For this review, take the finished solid that the model builds, in its own axes (mm). Face numbers are marked on the shaded views. Round coordinates to 2 decimals unless told otherwise and drop trailing zeros. Order: outer loops, then holes, each group sorted by start corner. A loop starts at its lowest first (then second) coordinate and runs counter-clockwise, first axis right, second up.
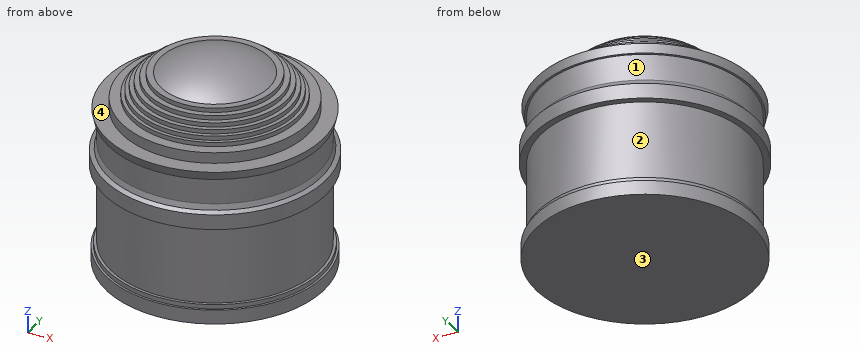
from build123d import *


with BuildPart() as f1:
    # F0 (on Front) → F1 (revolve)
    with BuildSketch(Plane.XZ):
        with BuildLine():
            Line((0, 76.2), (0, 38.1))
            Line((0, 38.1), (0, -76.2))
            Line((0, -76.2), (79.872511, -76.2))
            Line((79.872511, -76.2), (79.872511, -65.777272))
            Line((79.872511, -65.777272), (78.254335, -65.777272))
            Line((78.254335, -65.777272), (78.254335, -62.504791))
            Line((78.254335, -62.504791), (76.2, -62.504791))
            Line((76.2, -62.504791), (76.2, -4.198033))
            Line((76.2, -4.198033), (80.9625, -4.198033))
            Line((80.9625, -4.198033), (80.9625, 6.914467))
            Line((80.9625, 6.914467), (77.836014, 8.487052))
            Line((77.836014, 8.487052), (76.2, 12.349062))
            Line((76.2, 12.349062), (76.2, 31.75))
            Line((76.2, 31.75), (77.7875, 31.75))
            Line((77.7875, 31.75), (79.375, 38.1))
            Line((79.375, 38.1), (68.2625, 38.1))
            Line((68.2625, 38.1), (68.2625, 46.0375))
            Line((68.2625, 46.0375), (60.720578, 46.0375))
            Line((60.720578, 46.0375), (60.720578, 49.2125))
            Line((60.720578, 49.2125), (58.177056, 49.2125))
            Line((58.177056, 49.2125), (58.177056, 52.3875))
            Line((58.177056, 52.3875), (55.33525, 52.3875))
            Line((55.33525, 52.3875), (55.33525, 55.5625))
            Line((55.33525, 55.5625), (52.146415, 55.5625))
            Line((52.146415, 55.5625), (52.146415, 58.7375))
            Line((52.146415, 58.7375), (48.542209, 58.7375))
            Line((48.542209, 58.7375), (48.542209, 61.9125))
            Line((48.542209, 61.9125), (44.421643, 61.9125))
            Line((44.421643, 61.9125), (44.421643, 65.0875))
            Line((44.421643, 65.0875), (39.623949, 65.0875))
            ThreePointArc((39.623949, 65.0875), (20.576352, 73.369297), (0, 76.2))
        make_face()
    revolve(axis=Axis((0, 0, -19.05), (0, 0, -1)))


solid = f1.part
(1) Add section A-A on z = -35. Give the boundary of the cut face in (x, y).
(2) Clearance check with flat-ended pins moving along their axes: P1, Ø10, axis at x = 59.5, z = -18.5, coming from the -Y side; P2, Ø4, axis at x = 28.5, z = 25.5, coming from the +Y side; P3, Ø4, axis at x = -30.5, z = 4, coming from the -Y side. State where each tip first meets the part, or that it passes through.
(3) Wall thickness on L1, parallel to Z at x = -68, y = -29; L2, parallel to Z at x = 44, y = 34; L3, parallel to X at y = 32, z = 12.5: over which ranges is each line inside the solid? List them lowest first.
(4) Draft analysis for pull direction Z (two halves, no side actions). For the marked faces 1, 2, 3 and 4, state which applies: pulls with the +Z half, pulls with the -Z half, needs draft (parallel to the pull), parting line crosses it, or undercut.
Here are the results:
1. outline: circle Ø152.4 at (0, 0)
2. P1: stops at y = -53.26
2. P2: stops at y = 71.44
2. P3: stops at y = -75.78
3. L1: z = -76.2 to 38.1
3. L2: z = -76.2 to 52.39
3. L3: x = -69.16 to 69.16
4. face 1: undercut
4. face 2: undercut
4. face 3: pulls with the -Z half
4. face 4: pulls with the +Z half
